For this review, take the finished solid that the model builds, in its own axes (mm). A direction names the side the tool comes from. Give positions to 0.01 mm unless a question says otherwise; leave off trailing zeros. Order: outer loops, then holes, each group sorted by start corner. A loop starts at its lowest first (then second) coordinate and runs counter-clockwise, first axis right, second up.
Item 1: For P1, Ø1, axis at x = -22, y = 5.5, coming from the -Z side; P2, Ø6, axis at x = 0, z = -3.5, coming from the +Y side; P3, Ø4, axis at y = 13, z = 22.5, coming from the +X side, all flat-tipped, find the tip position at first contact; note any pin that passes through.
Item 2: For probe 1 along X at (y, z) = (18.55, 0); probe 2 along X at (y, z) = (5.25, 12); probe 3 along Y at (x, z) = (-28, 22.5), list the stretches that pass through material, from the lowest coordinate up.
Item 3: Consider section B-B (y = 14.25). Give the boundary of the cut face in (x, z).
Item 4: Consider section A-A (y = 3). Give the boundary of the cut face in (x, z).
Item 5: Machinability: for faces 1 (the flat face through (0, 20, -14)), 2 (the flat face through (-0.14, 17.5, -0.14)), which of the approach directions +Z, -Z, +X, -X, +Y, -Y give a long, thin tool a straight path to every point of the face, cutting with its end or side? Answer none if there is none.
Item 6: The part is to be moulded in two halves that separate along X. For faces 3 (the flat face through (0, 10, 20)), 4 (the cylindrical face through (-2.25, 18.77, -10)), 5 (the flat face through (-1, 0, -1)), say which applies: released by +X, released by -X, zero draft, split by the parting line, or undercut.
```python
from build123d import *

# Parameters (mm, degrees)
BOSS_EXTRUDE1_DEPTH = 20
SKETCH3_R           = 10.25
CUT_EXTRUDE1_DEPTH  = 2.5
FILLET1_R           = 10


with BuildPart() as part:
    # Sketch1 → Boss-Extrude1 (new body)
    with BuildSketch(Plane(origin=(0, 0, 0), x_dir=(1, 0, 0), z_dir=(0, 1, 0))):
        with BuildLine():
            Line((0, -40), (0, 0))
            Line((0, 0), (20, -34.641016151))
            ThreePointArc((20, -34.641016151), (34.641016151, -20), (40, 0))
            ThreePointArc((40, 0), (-28.284271247, 28.284271247), (0, -40))
        make_face()
    extrude(amount=BOSS_EXTRUDE1_DEPTH)

    # Sketch3 → Cut-Extrude1 (cut)
    with BuildSketch(Plane(origin=(0, 20, 0), x_dir=(1, 0, 0), z_dir=(0, 1, 0))):
        Circle(SKETCH3_R)
    extrude(amount=-CUT_EXTRUDE1_DEPTH, mode=Mode.SUBTRACT)

    # Fillet1
    fillet1_edges = [part.edges().sort_by_distance(p)[0] for p in [
        (-10.352761804, 20, -38.637033052),
    ]]
    fillet(fillet1_edges, radius=FILLET1_R)


solid = part.part
```
Resolved:
1. P1: stops at z = -33.73
1. P2: stops at y = 17.5
1. P3: stops at x = 33.96
2. probe 1: x = -35.19 to -10.25, 10.25 to 35.19
2. probe 2: x = -38.16 to 0, 6.93 to 38.16
2. probe 3: y = 0 to 18.06
3. outline: (0, 0) - (0, 39.05) arc R39.05 ccw (long way) to (19.53, 33.82) - close
4. outline: (0, 0) - (0, 40) arc R40 ccw (long way) to (20, 34.64) - close
5. face 1: +Z, -Z, +X, -X, +Y
5. face 2: +Y
6. face 3: undercut
6. face 4: undercut
6. face 5: zero draft
